Solid Edge part; units mm, degrees
sketch "Sketch1" plane through (0, 0, 0) normal (0, 0, 1) x (1, 0, 0)
  line L0 (30, -4) -> (-30, -4)
  line L1 (-30, -4) -> (-30, 4)
  line L2 (-30, 4) -> (30, 4)
  line L3 (30, 4) -> (30, -4)
extrude "Protrusion1" add sketch "Sketch1" along normal mid plane 5
sketch "Sketch2" plane through (0, 0, 0) normal (0, -1, 0) x (1, 0, 0)
  circle A0 centre (0, 0) radius 1
extrude "ExtrudedCutout_1" cut sketch "Sketch2" along normal mid plane 38.2729
Can you work these out from the model? Positions are in its coordinate system, mm. Round coordinates to 2 decimals unless told otherwise and drop trailing zeros. Loops run counter-clockwise (first coordinate to the right, second up) from the corner with the lowest first, then second, coordinate; pieces in that order, holes last. Notation, with made-up numbers: M 82,-33.5 L 86,-33.5 A12 cw 86,-20.5 Z; hole C 65,26 d1. An arc over 180 degrees is marked long. Write item = value, one per line. Start each with the question number.
(1) If we mould it in two halves opening along Z, with no side actions, what happens to faces 1 (the face through (0, 0, -2.5)), 2 (the face through (0.4, -4, -1.1)), 3 (the face through (0, 0, -1))? For each: released by +Z, released by -Z, zero draft, split by the parting line, or undercut.
(2) I need wall thicknesses on line 1 along X through (y, z) = (1, 0); line 2 along Z through (x, y) = (0, 0.25); line 3 along X through (y, z) = (0.75, 0.9). Which ranges of each line are inside material? Lowest first, please.
(3) Suppose I cut it at A-A on z = 0. Write out the boundary of the cut face in (x, y), plus the area to 3 significant figures.
(4) Suppose I cut it at B-B on x = 0. Write out the boundary of the cut face in (y, z), plus the area to 3 significant figures.
Answer block:
q1.face_1 = released by -Z
q1.face_2 = zero draft
q1.face_3 = undercut
q2.line_1 = -30 to -1, 1 to 30
q2.line_2 = -2.5 to -1, 1 to 2.5
q2.line_3 = -30 to -0.44, 0.44 to 30
q3.outline = M -30,-4 L -1,-4 L -1,4 L -30,4 Z; M 1,-4 L 30,-4 L 30,4 L 1,4 Z
q3.area = 464 mm²
q4.outline = M -4,-2.5 L 4,-2.5 L 4,-1 L -4,-1 Z; M -4,1 L 4,1 L 4,2.5 L -4,2.5 Z
q4.area = 24.0 mm²
